The model under review builds one solid part; all positions refer to its coordinate system, in mm. Face numbers are marked on the shaded views. Give positions to 0.01 mm unless a question says otherwise; leave off trailing zeros. Order: outer loops, then holes, each group sorted by start corner. A loop starts at its lowest first (then second) coordinate and runs counter-clockwise, first axis right, second up. Notation, with made-up numbers: (54, -30.5) - (85, -30.5) arc R8 ccw to (85, -26.5) - close; hole circle Ø2 at (-29, 15). An arc over 180 degrees is marked (long way). Put each result on its own line as item: value.
```python
from build123d import *

# Parameters (mm, degrees)
SKETCH1_W           = 81.5
SKETCH1_H           = 102.5
BOSS_EXTRUDE1_DEPTH = 6
SKETCH2_R           = 1.5
CUT_EXTRUDE1_DEPTH  = 7
SKETCH7_W           = 79.5
SKETCH7_H           = 100.5
CUT_EXTRUDE3_DEPTH  = 1.85
SKETCH8_W           = 79.5
SKETCH8_H           = 100.5
SKETCH8_R           = 2.5
CUT_EXTRUDE4_DEPTH  = 2.4
FILLET1_R           = 1
CHAMFER1_SIZE       = 0.25


with BuildPart() as part:
    # Sketch1 → Boss-Extrude1 (new body)
    with BuildSketch(Plane(origin=(0, 0, 0), x_dir=(1, 0, 0), z_dir=(0, 1, 0))):
        Rectangle(SKETCH1_W, SKETCH1_H)
    extrude(amount=BOSS_EXTRUDE1_DEPTH)

    # Sketch2 → Cut-Extrude1 (cut, through all)
    with BuildSketch(Plane(origin=(0, 6, 0), x_dir=(1, 0, 0), z_dir=(0, 1, 0))):
        with Locations((-35.5, -46)):
            Circle(SKETCH2_R)
        with Locations((-35.5, 40)):
            Circle(SKETCH2_R)
        with Locations((22.5, -46)):
            Circle(SKETCH2_R)
        with Locations((22.5, 40)):
            Circle(SKETCH2_R)
    extrude(amount=-CUT_EXTRUDE1_DEPTH, mode=Mode.SUBTRACT)

    # Sketch7 → Cut-Extrude3 (cut)
    with BuildSketch(Plane(origin=(0, 6, 0), x_dir=(1, 0, 0), z_dir=(0, 1, 0))):
        Rectangle(SKETCH7_W, SKETCH7_H)
    extrude(amount=-CUT_EXTRUDE3_DEPTH, mode=Mode.SUBTRACT)

    # Sketch8 → Cut-Extrude4 (cut)
    with BuildSketch(Plane(origin=(0, 4.15, 0), x_dir=(1, 0, 0), z_dir=(0, 1, 0))):
        Rectangle(SKETCH8_W, SKETCH8_H)
        with Locations((-35.5, 40)):
            Circle(SKETCH8_R, mode=Mode.SUBTRACT)
        with Locations((22.5, 40)):
            Circle(SKETCH8_R, mode=Mode.SUBTRACT)
        with Locations((-35.5, -46)):
            Circle(SKETCH8_R, mode=Mode.SUBTRACT)
        with Locations((22.5, -46)):
            Circle(SKETCH8_R, mode=Mode.SUBTRACT)
    extrude(amount=-CUT_EXTRUDE4_DEPTH, mode=Mode.SUBTRACT)

    # Fillet1
    fillet1_edges = [part.edges().sort_by_distance(p)[0] for p in [
        (-39.75, 3.875, 50.25),
        (-39.75, 3.875, -50.25),
        (39.75, 3.875, -50.25),
        (39.75, 3.875, 50.25),
        (-40.75, 3, 51.25),
        (-40.75, 3, -51.25),
        (40.75, 3, -51.25),
        (40.75, 3, 51.25),
    ]]
    fillet(fillet1_edges, radius=FILLET1_R)

    # Chamfer1
    chamfer1_edges = [part.edges().sort_by_distance(p)[0] for p in [
        (-37, 4.15, 46),
        (21, 4.15, -40),
        (21, 4.15, 46),
        (-37, 4.15, -40),
    ]]
    chamfer(chamfer1_edges, length=CHAMFER1_SIZE)


solid = part.part
```
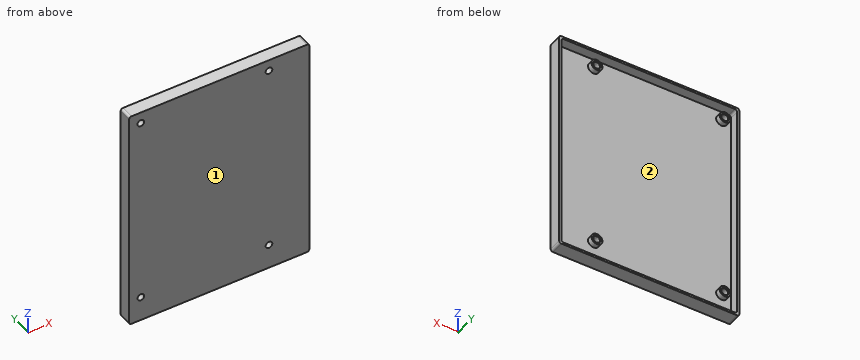
(1) Take a section at D-D, the plane x = 11.5. Write out the cut boundary in (y, z).
The answers:
outline: (0, -51.25) - (6, -51.25) - (6, -50.25) - (1.75, -50.25) - (1.75, 50.25) - (6, 50.25) - (6, 51.25) - (0, 51.25) - close
(2) Clearance check with flat-ended pins moving along their axes: pin 1 Ø1.5 at (x, z) = (22, -39) entering from +Y; pin 2 Ø24 at (x, z) = (12.5, 19.5) entering from +Y; pin 3 Ø1.5 at (x, z) = (-35.5, -40) entering from +Y. State where each tip first meets the part, or that it passes through.
The answers:
pin 1: y = 4.15
pin 2: y = 1.75
pin 3: through
(3) Wall thickness on L1, parallel to X at y = 1.65, z = 46; L2, parallel to Z at x = -35.5, y = 3.15; L3, parallel to X at y = 2.6, z = -40: over which ranges is each line inside the solid? List them lowest first.
The answers:
L1: -40.75 to -37, -34 to 21, 24 to 40.75
L2: -51.25 to -50.25, -42.5 to -41.5, -38.5 to -37.5, 43.5 to 44.5, 47.5 to 48.5, 50.25 to 51.25
L3: -40.75 to -39.75, -38 to -37, -34 to -33, 20 to 21, 24 to 25, 39.75 to 40.75
(4) Take a section at A-A, the plane x = -35.5. Write out the cut boundary in (y, z).
The answers:
outline: (0, -51.25) - (6, -51.25) - (6, -50.25) - (1.75, -50.25) - (1.75, -42.5) - (4.15, -42.5) - (4.15, -41.75) - (3.9, -41.5) - (0, -41.5) - close; (0, -38.5) - (3.9, -38.5) - (4.15, -38.25) - (4.15, -37.5) - (1.75, -37.5) - (1.75, 43.5) - (4.15, 43.5) - (4.15, 44.25) - (3.9, 44.5) - (0, 44.5) - close; (0, 47.5) - (3.9, 47.5) - (4.15, 47.75) - (4.15, 48.5) - (1.75, 48.5) - (1.75, 50.25) - (6, 50.25) - (6, 51.25) - (0, 51.25) - close
(5) Take a section at B-B, the plane z = 46. Write out the cut boundary in (x, y), then the cut area to 3 significant figures.
The answers:
outline: (-40.75, 0) - (-37, 0) - (-37, 3.9) - (-37.25, 4.15) - (-38, 4.15) - (-38, 1.75) - (-39.75, 1.75) - (-39.75, 6) - (-40.75, 6) - close; (-34, 0) - (21, 0) - (21, 3.9) - (20.75, 4.15) - (20, 4.15) - (20, 1.75) - (-33, 1.75) - (-33, 4.15) - (-33.75, 4.15) - (-34, 3.9) - close; (24, 0) - (40.75, 0) - (40.75, 6) - (39.75, 6) - (39.75, 1.75) - (25, 1.75) - (25, 4.15) - (24.25, 4.15) - (24, 3.9) - close
area: 150 mm^2
(6) The part is to be moulded in two halves that separate along X. For the marked faces 1 and 2, say which applies: pulls with the +X half, pulls with the -X half, needs draft (parallel to the pull), parting line crosses it, or undercut.
The answers:
face 1: needs draft
face 2: undercut
(7) Take a section at C-C, the plane z = -31.5. Write out the cut boundary in (x, y).
The answers:
outline: (-40.75, 0) - (40.75, 0) - (40.75, 6) - (39.75, 6) - (39.75, 1.75) - (-39.75, 1.75) - (-39.75, 6) - (-40.75, 6) - close
